Source: CAD feature listing. Evaluate the final solid. Frame: model axes, mm. A direction names the side the tool comes from. Coordinates: 2 decimals unless noted, no trailing zeros. Loops run counter-clockwise (first coordinate to the right, second up) from the corner with the lowest first, then second, coordinate; pieces in that order, holes last.
Autodesk Inventor part; units mm, degrees
ref_plane "Work Plane1" through (30.1625, 0, 0) normal (0, 0, -1) x (1, 0, 0)
ref_plane "YZ Plane" through (0, 0, 0) normal (1, 0, 0) x (0, 1, 0)
ref_plane "XZ Plane" through (0, 0, 0) normal (0, 1, 0) x (-1, 0, 0)
sketch "Эскиз1" plane through (0, 0, 0) normal (0, 0, 1) x (1, 0, 0)
  line L0 (-2.4, 0) -> (10, 0)
  line L1 (10, 0) -> (10, 1.75)
  line L2 (10, 1.75) -> (1.2, 1.75)
  line L3 (1.2, 1.75) -> (0.8318, 1.5876)
  line L4 (0.8318, 1.5876) -> (0, 1.5876)
  line L5 (0, 1.5876) -> (0, 3)
  line L6 (-4.88, 0) -> (12.48, 0)
  line L7 (0, -0.6) -> (0, 3.6)
  line L8 (-2.4, 0) -> (-2.4, 2.79)
  line L9 (0, 3) -> (-2.4, 2.79)
  line L10 (1.2, 1.75) -> (0, 1.75) construction
  dimension "d0" = 10
  dimension "d1" = 8.8
  dimension "d2" = 0.3682
  dimension "d3" = 2.4
  dimension "d4" = 3.5
  dimension "d5" = 3.1752
  dimension "d9" = 6
  dimension "d10" = 5
revolve "Базовый элемент" add sketch "Эскиз1" angle 360 about axis through (-2.4, 0, 0) along (1, 0, 0)
sketch "Эскиз2" plane through (-2.4, 0, 0) normal (-1, 0, 0) x (0, 0, 1)
  circle A0 centre (0, 0) radius 3
  line L0 (0, 0) -> (0, 2.79)
  line L1 (-3, 0.5) -> (3, 0.5)
  line L2 (3, 0.5) -> (3, -0.5)
  line L3 (3, -0.5) -> (-3, -0.5)
  line L4 (-3, -0.5) -> (-3, 0.5)
  line L5 (-3, 0) -> (3, 0) construction
  line L6 (0, 0.5) -> (0, -0.5) construction
  dimension "d11" = 1
  dimension "d12" = 6
fillet "Сопряжение1" radius 0.1 1 edges at (-2.4, -2.79, 0)
extrude "Паз" cut sketch "Эскиз2" against normal blind 1 contours A0 L3 L1 | L2 L3 A0 | A0 L1 L2 | A0 L4 L1 | L3 L4 A0
thread "Резьба"
chamfer "Фаска1" distance 0.3248 distance2 0.3682 1 edges at (10, -1.75, 0) measured on face at (10, 0.4197, 0.5264)
ref_plane "Work Plane1" through (30.1625, 0, 0) normal (0, 0, -1) x (1, 0, 0)
equation "\"d11\" = SBR"
equation "\"d12\" = KOD"
equation "\"d14\" = RR"
equation "\"d19\" = STI"
equation "\"d15\" = GEL"
equation "\"d17\" = -0.5 * SPD + 0.5 * GD"
equation "\"d0\" = NLG"
equation "\"d1\" = GEL"
equation "\"d3\" = KOH"
equation "\"d4\" = GD"
equation "\"d5\" = BDM"
equation "\"d9\" = KOD"
equation "\"d10\" = KEWI"
equation "\"GD\" = 3.5"
equation "\"NLG\" = 10"
equation "\"GEL\" = 8.8"
equation "\"KOD\" = 6"
equation "\"KOH\" = 2.4"
equation "\"GAL\" = 0.61345 * PTC"
equation "\"SPD\" = 2.85048"
equation "\"BDM\" = 3.17524"
equation "\"GUL\" = 0.61345 * PTC"
equation "\"RR\" = 0.1"
equation "\"SBR\" = 1"
equation "\"STI\" = 1"
equation "\"KEWI\" = 5deg"
equation "\"PTC\" = 0.6"
equation "\"THREADDIA\" = 3.5"
equation "\"TOA\" = 30deg"
equation "\"NND\" = 3.5"
equation "\"GD1\" = THREADDIA - 1.2269 * PTC"
properties part number "DIN 84 - M3,5 x 10" material "Сталь, мягкая"
Q1. Section B-B, the plane y = 0. Return the cut outline in (x, z).
Q2. Contact query for flat-ended pins moving along their axis: pin 1 Ø0.8 at (x, z) = (-2, -0.5) entering from +Y; pin 2 Ø0.5 at (x, z) = (-2, -0.5) entering from -Y; pin 3 Ø0.8 at (y, z) = (0, -1) entering from -X. Output: stop coordinate, or through.
Q3. Section A-A, the plane z = 0. Return the cut outline in (x, y), plus the area to 3 significant figures.
Q4. Access query for faces 1 (the cylindrical face through (5.357, 1.617, 0.67)), 2 (the flat face through (-2, 0.5, 0)), 3 (the cylindrical face through (0.41, -0.207, -1.574)), 4 (the flat face through (-2.4, -1, 0)). Directions: +Z, -Z, +X, -X, +Y, -Y. A direction counts if a zero-diameter tool reaches every point of the face in a straight line with its end or side. Return the directions, or none.
Q5. Section C-C, the plane x = 2.5. Return the cut outline in (y, z).
Q6. Section D-D, the plane x = 0.5. Return the cut outline in (y, z), plus the area to 3 significant figures.
Q7. Draft query along Y for faces 5 (the flat face through (-1.4, 0, 0)), 6 (the flat face through (10, 0, 0)), 7 (the conical face through (-1.395, 1.328, -2.553)). Return one class per face: +Y half, -Y half, draft (parallel to the pull), parting line (faces both ways), or undercut.
Q8. Line query: line 1 along X through (y, z) = (-0.7, -2.2); line 2 along X through (y, z) = (0.1, -2.1); line 3 along Z through (x, y) = (7.5, 0.05). Output: solid intervals per line, ascending.
Derived:
1. outline: (-1.4, -2.88) - (0, -3) - (0, -1.59) - (0.83, -1.59) - (1.2, -1.75) - (9.63, -1.75) - (10, -1.43) - (10, 1.43) - (9.63, 1.75) - (1.2, 1.75) - (0.83, 1.59) - (0, 1.59) - (0, 3) - (-1.4, 2.88) - close
2. pin 1: stops at y = 2.84
2. pin 2: stops at y = -2.82
2. pin 3: stops at x = -1.4
3. outline: (-2.4, -2.7) arc R0.1 ccw to (-2.31, -2.8) - (0, -3) - (0, -1.59) - (0.83, -1.59) - (1.2, -1.75) - (9.63, -1.75) - (10, -1.43) - (10, 1.43) - (9.63, 1.75) - (1.2, 1.75) - (0.83, 1.59) - (0, 1.59) - (0, 3) - (-2.31, 2.8) arc R0.1 ccw to (-2.4, 2.7) - (-2.4, 0.5) - (-1.4, 0.5) - (-1.4, -0.5) - (-2.4, -0.5) - close
3. area: 47.4 mm2
4. face 1: +X
4. face 2: +Z, -Z, -X
4. face 3: none
4. face 4: +Z, -Z, -X, +Y, -Y
5. outline: circle Ø3.5 at (0, 0)
6. outline: circle Ø3.18 at (0, 0)
6. area: 7.92 mm2
7. face 5: undercut
7. face 6: draft
7. face 7: parting line
8. line 1: x = -2.4 to 0
8. line 2: x = -1.4 to 0
8. line 3: z = -1.75 to 1.75
